```python
from build123d import *

# Parameters (mm, degrees)
SKETCH2_R            = 76.2
SKETCH2_R_2          = 50.8
BOSS_EXTRUDE7_DEPTH  = 127
BOSS_EXTRUDE8_DEPTH  = 101.6
SKETCH2_12_W         = 304.8
SKETCH2_12_H         = 50.8
BOSS_EXTRUDE9_DEPTH  = 152.4
BOSS_EXTRUDE10_DEPTH = 25.4


with BuildPart() as part:
    # Sketch2 → Boss-Extrude7 (new body)
    with BuildSketch(Plane.XY):
        Circle(SKETCH2_R)
        Circle(SKETCH2_R_2, mode=Mode.SUBTRACT)
    extrude(amount=BOSS_EXTRUDE7_DEPTH)

    # Sketch2_11 → Boss-Extrude8 (add)
    with BuildSketch(Plane.XY):
        with BuildLine():
            ThreePointArc((12.7, -75.134213245), (0, -76.2), (-12.7, -75.134213245))
            Line((-12.7, -75.134213245), (-12.7, -203.2))
            Line((-12.7, -203.2), (12.7, -203.2))
            Line((12.7, -203.2), (12.7, -75.134213245))
        make_face()
    extrude(amount=BOSS_EXTRUDE8_DEPTH)

    # Sketch2_12 → Boss-Extrude9 (add)
    with BuildSketch(Plane.XY):
        with Locations((0, -228.6)):
            Rectangle(SKETCH2_12_W, SKETCH2_12_H)
    extrude(amount=BOSS_EXTRUDE9_DEPTH)

    # Sketch2_13 → Boss-Extrude10 (add)
    with BuildSketch(Plane.XY):
        with BuildLine():
            ThreePointArc((-12.7, -75.134213245), (-58.198711326, -49.186888497), (-76.2, 0))
            Line((-76.2, 0), (-152.4, -203.2))
            Line((-152.4, -203.2), (-12.7, -203.2))
            Line((-12.7, -203.2), (-12.7, -75.134213245))
        make_face()
        with BuildLine():
            Line((152.4, -203.2), (76.2, 0))
            ThreePointArc((76.2, 0), (58.198711326, -49.186888497), (12.7, -75.134213245))
            Line((12.7, -75.134213245), (12.7, -203.2))
            Line((12.7, -203.2), (152.4, -203.2))
        make_face()
    extrude(amount=BOSS_EXTRUDE10_DEPTH)


solid = part.part
```
Here's how the part is built. I have some questions about the finished solid (model axes, mm). A direction names the side the tool comes from. Give positions to 0.01 mm unless a question says otherwise; leave off trailing zeros. Order: outer loops, then holes, each group sorted by start corner. A loop starts at its lowest first (then second) coordinate and runs counter-clockwise, first axis right, second up. Notation, with made-up numbers: (79.5, 53) - (112.5, 53) arc R32 ccw to (112.5, 84) - close; hole circle Ø4 at (67, 26.5). An arc over 180 degrees is marked (long way). Answer as a JSON object with one key per item and string values. Group by question number.
Item 1: If we section it at D-D on y = -7: Please give me the cut outline in (x, z) (3 decimals).
Item 2: Please list where these lines run through material, in increasing order: probe 1 along Y at (x, z) = (-1, 31.5); probe 2 along Y at (x, z) = (-19, 83); probe 3 along Z at (x, y) = (103.5, -178).
Item 3: For P1, Ø6, axis at y = -191.5, z = 103.5, coming from the -X side; P2, Ø1.5, axis at x = 9.5, y = -118.5, coming from the +Z side; P3, Ø6, axis at y = 6.5, z = 75, coming from the -X side, each with a flat end and sliding along its axis, tell me the tip position at first contact or that it passes through.
Item 4: If we section it at A-A on z = 116: Please give me the cut outline in (x, y), and give its area (3 significant figures).
Item 5: If we mould it in two halves opening along X, with no side actions, what happens to faces 1 (the cylindrical face through (-11.012, -49.592, 62.611)), 2 (the flat face through (0, -138, 101.6)), 3 (the flat face through (12.7, -140, 63)), 4 (the flat face through (-12.7, -138, 63))? For each: pulls with the +X half, pulls with the -X half, needs draft (parallel to the pull), parting line crosses it, or undercut.
Item 6: If we section it at C-C on z = 10: Please give me the cut outline in (x, y).
Item 7: Which directions (+Z, -Z, +X, -X, +Y, -Y) give clear straight access to the entire face, cutting with the end or side of a thin tool? Please do faces 5 (the flat face through (-2, -203.2, 102)), 6 (the flat face through (66, -123, 25.4)), 7 (the flat face through (-68, -123, 25.4)), 8 (the flat face through (16, -50, 127)).
Item 8: If we section it at B-B on x = 0: Please give me the cut outline in (y, z), and give its area (3 significant figures).
Result set:
{
 "1": {"outline": "(-78.825, 0) - (-50.315, 0) - (-50.315, 127) - (-75.878, 127) - (-75.878, 25.4) - (-78.825, 25.4) - close; (50.315, 0) - (78.825, 0) - (78.825, 25.4) - (75.878, 25.4) - (75.878, 127) - (50.315, 127) - close"},
 "2": {"probe 1": "-254 to -50.79, 50.79 to 76.19", "probe 2": "-254 to -203.2, -73.79 to -47.11, 47.11 to 73.79", "probe 3": "0 to 25.4"},
 "3": {"P1": "x = -12.7", "P2": "z = 101.6", "P3": "x = -76.12"},
 "4": {"outline": "(-152.4, -254) - (152.4, -254) - (152.4, -203.2) - (-152.4, -203.2) - close; circle Ø152.4 at (0, 0); hole circle Ø101.6 at (0, 0)", "area": "25,600 mm²"},
 "5": {"face 1": "undercut", "face 2": "needs draft", "face 3": "pulls with the +X half", "face 4": "pulls with the -X half"},
 "6": {"outline": "(-152.4, -254) - (152.4, -254) - (152.4, -203.2) - (76.2, 0) arc R76.2 ccw to (-76.2, 0) - (-152.4, -203.2) - close; hole circle Ø101.6 at (0, 0)"},
 "7": {"face 5": "+Z", "face 6": "+Z, +X", "face 7": "+Z, -X", "face 8": "+Z, +X, -X, +Y"},
 "8": {"outline": "(-254, 0) - (-50.8, 0) - (-50.8, 127) - (-76.2, 127) - (-76.2, 101.6) - (-203.2, 101.6) - (-203.2, 152.4) - (-254, 152.4) - close; (50.8, 0) - (76.2, 0) - (76.2, 127) - (50.8, 127) - close", "area": "27,100 mm²"}
}
